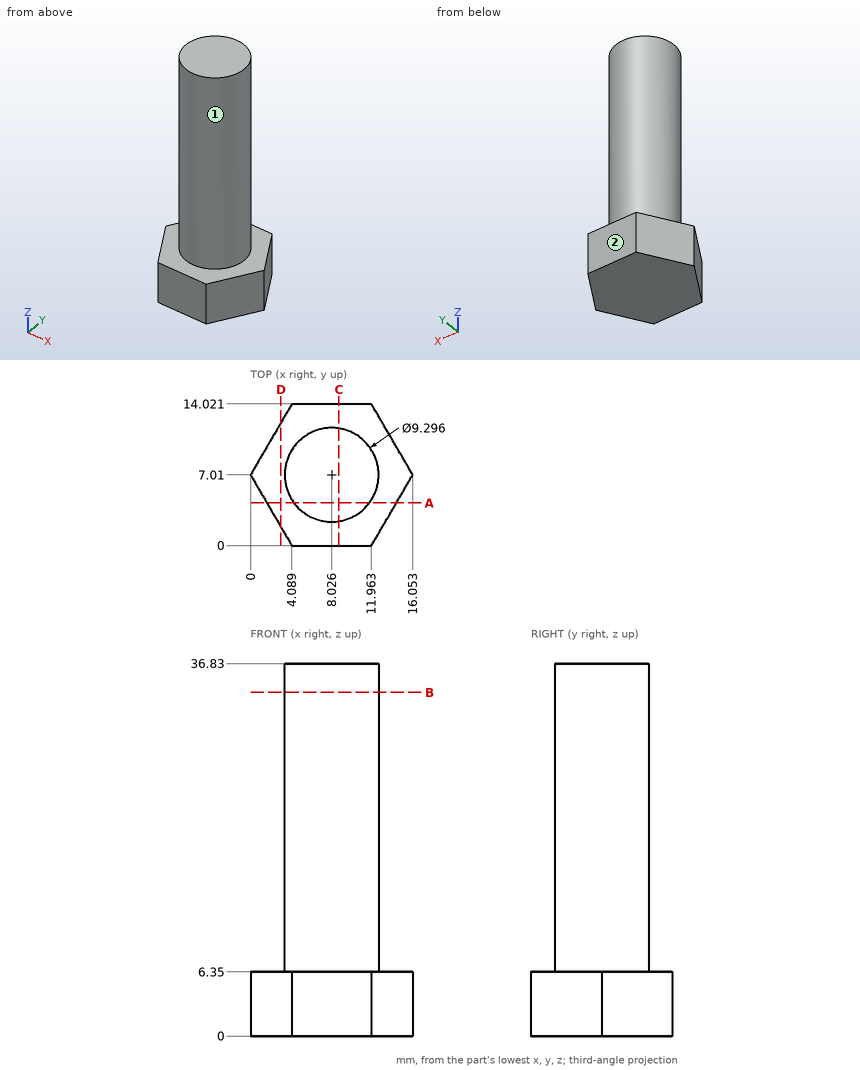
Job drawing, mm, ordinate dimensions from the low corner. One solid piece. A direction names the side the tool comes from. Give positions to 0.01 mm unless a question says otherwise; leave off trailing zeros. Write each loop counter-clockwise with the first axis right and the second up, starting at its lowest first coordinate (ties: lowest second). Pieces come first, ordered by that corner, then holes. Notation, with made-up numbers: M 74.5,49.25 L 88.5,49.25 A15 ccw 88.5,59.25 Z; hole C -7,-17 d6. An arc over 180 degrees is marked long. Put each result on its own line as item: value. Start each with the question number.
(1) Band-saw the part on C-C, the plane x = 8.75. Write the cut outline in (y, z).
(2) Which spindle directions (+Z, -Z, +X, -X, +Y, -Y) get a long thin tool onto all of the face, cutting with end or side? Do the marked faces 1 and 2. Say none if no direction does.
(3) Flat gauge pins, fed straight in: pin 1 Ø1.5 at (y, z) = (2, 6.5) entering from -X (1 decimal); pin 2 Ø5 at (y, z) = (3.5, 27) entering from -X; pin 3 Ø2 at (x, y) = (12.5, 12) entering from +Z. Where does each tip first touch, or does it go through?
(4) Band-saw the part on B-B, the plane z = 34. Write the cut outline in (x, y).
(5) Probe L1, parallel to Z at x = 2.75, y = 11; L2, parallel to Y at x = 8.25, z = 29; L3, parallel to Y at x = 14.75, z = 5.5 (1 decimal). List the from-to ranges inside material, lowest first.
(6) Band-saw the part on D-D, the plane x = 3. Write the cut outline in (y, z).
(7) Band-saw the part on A-A, the plane y = 4.25. Write the cut outline in (x, z).
Response values:
1. outline: M 0,0 L 14.02,0 L 14.02,6.35 L 11.6,6.35 L 11.6,36.83 L 2.42,36.83 L 2.42,6.35 L 0,6.35 Z
2. face 1: +Z
2. face 2: +Z, -Z, +X, -X, +Y
3. pin 1: stops at x = 2.5
3. pin 2: stops at x = 3.49
3. pin 3: stops at z = 6.35
4. outline: C 8.03,7.01 d9.3
5. L1: z = 0 to 6.35
5. L2: y = 2.37 to 11.65
5. L3: y = 4.8 to 9.2
6. outline: M 1.87,0 L 12.15,0 L 12.15,6.35 L 1.87,6.35 Z
7. outline: M 1.61,0 L 14.44,0 L 14.44,6.35 L 11.77,6.35 L 11.77,36.83 L 4.29,36.83 L 4.29,6.35 L 1.61,6.35 Z
